from build123d import *

# Parameters (mm, degrees)
F1_DEPTH = 1.85
F3_DEPTH = 2


with BuildPart() as f1:
    # F0 (on Front) → F1 (new body)
    with BuildSketch(Plane.XZ):
        with BuildLine():
            ThreePointArc((10.181424, 35.10782), (15.688682, 34.328624), (18.692279, 39.010018))
            ThreePointArc((18.692279, 39.010018), (12.611069, 44.075129), (8.729038, 37.178296))
            ThreePointArc((8.729038, 37.178296), (9.326157, 36.052516), (10.181424, 35.10782))
        make_face()
        with BuildLine():
            ThreePointArc((10.181424, 35.10782), (9.326157, 36.052516), (8.729038, 37.178296))
            Line((8.729038, 37.178296), (7.740627, 36.03068))
            Line((7.740627, 36.03068), (9.598273, 34.43074))
            Line((9.598273, 34.43074), (10.181424, 35.10782))
        make_face()
        Polygon((9.598273, 34.43074), (7.740627, 36.03068), (4.324033, 38.973298), (-5.589027, 38.973298), (-12.540483, 30.902152), (-9.313422, 28.122773), (-3.636302, 34.714323), (0, 34.714323), (-15.893627, 16.260666), (-28.178568, 16.260666), (-28.178568, 8.741623), (-26.115432, 8.741623), (-26.115432, 12.00169), (-12.288238, 12.00169), (-6.393013, 18.846476), (0.451773, 12.951251), (-4.339739, 3.737698), (0, 0), (3.78513, 0), (3.78513, 2.063135), (0.915639, 2.063135), (0, 2.85175), (6.379701, 15.119216), (0.429039, 20.244357), (8.569453, 29.69597), (15.320196, 23.881742), (22.271652, 31.952888), (19.044591, 34.732267), (14.872513, 29.888182), align=None)
    extrude(amount=F1_DEPTH)

    # F2 (on face) → F3 (join)
    with BuildSketch(Plane.XZ.offset(1.85)):
        Polygon((-4.339739, 3.737698), (0, 0), (3.78513, 0), (3.78513, 2.063135), (0.915639, 2.063135), (-3.315463, 5.707268), align=None)
    extrude(amount=F3_DEPTH)


solid = f1.part
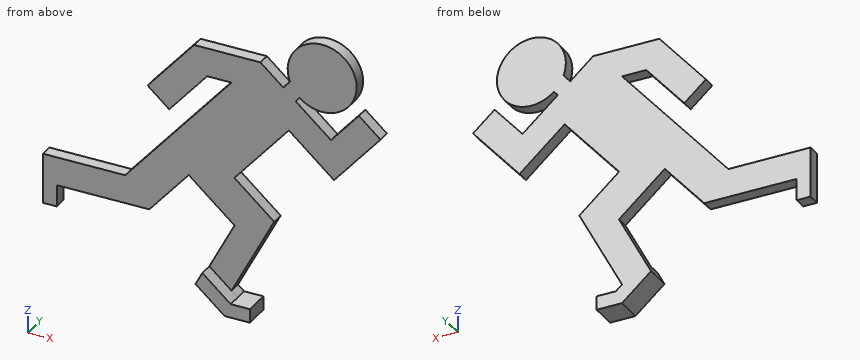
Geometry check sheet. Reference: the model listing, model coordinates, mm. Give positions to 0.01 mm unless a question says otherwise; leave off trailing zeros. Loops run counter-clockwise (first coordinate to the right, second up) from the corner with the lowest first, then second, coordinate; pieces in that order, holes last.
(1) Depth check by flat-ended pin: pin 1 Ø2 at (x, z) = (-3.5, 33) entering from +Y; pin 2 Ø0.9 at (x, y) = (-27, -0.5) entering from -Z; pin 3 Ø1.5 at (x, y) = (-2, -1) entering from +Z; pin 4 Ø1.5 at (x, y) = (-2, -1.5) entering from -Z. Enter the tip coordinate at first touch or a pass-through.
From the geometry:
pin 1: passes through
pin 2: stops at z = 8.74
pin 3: stops at z = 38.97
pin 4: stops at z = 1.08
(2) Section check B-B on x = -11.5. Record the cut outline in (y, z).
From the geometry:
outline: (-1.85, 12.92) - (0, 12.92) - (0, 21.36) - (-1.85, 21.36) - close; (-1.85, 30.01) - (0, 30.01) - (0, 32.11) - (-1.85, 32.11) - close
(3) Section check D-D on x = -2.5. Record the cut outline in (y, z).
From the geometry:
outline: (-3.85, 2.15) - (0, 2.15) - (0, 7.28) - (-1.85, 7.28) - (-1.85, 5) - (-3.85, 5) - close; (-1.85, 15.49) - (0, 15.49) - (0, 31.81) - (-1.85, 31.81) - close; (-1.85, 34.71) - (0, 34.71) - (0, 38.97) - (-1.85, 38.97) - close
(4) Section check A-A on z = 38. Record the cut outline in (x, y).
From the geometry:
outline: (-6.43, -1.85) - (5.45, -1.85) - (5.45, 0) - (-6.43, 0) - close; (8.49, -1.85) - (18.59, -1.85) - (18.59, 0) - (8.49, 0) - close
(5) Thickness scan on L1, parallel to X at y = -1.65, z = 32; L2, parallel to X at y = -1.8, z = 34.5; L3, parallel to X at y = -1.6, z = 26. Record the ranges inside material, lowest first.
From the geometry:
L1: x = -11.59 to -5.97, -2.34 to 12.42, 16.69 to 22.22
L2: x = -9.44 to -3.82, -0.18 to 9.66, 11.06 to 16.03, 18.84 to 19.31
L3: x = -7.51 to 5.39, 12.86 to 17.14
